from build123d import *

# Parameters (mm, degrees)
F0_R      = 25.4
F1_DEPTH  = 76.2
F2_R      = 9.525
F3_DEPTH  = 19.05
F4_R      = 5.08
F5_SIZE   = 1.27
F6_W      = 19.05
F6_H      = 19.05
F7_DEPTH  = 19.05
F8_R      = 6.931889
F9_DEPTH  = 9.525
F10_R     = 4.338824
F11_DEPTH = 25.4
F12_SIZE  = 1.27
F13_R     = 1.27


with BuildPart() as f1:
    # F0 (on Top) → F1 (new body)
    with BuildSketch(Plane.XY):
        Circle(F0_R)
    extrude(amount=F1_DEPTH)

    # F2 (on face) → F3 (join)
    with BuildSketch(Plane(origin=(0, 0, 0), x_dir=(1, 0, 0), z_dir=(0, 0, -1))):
        Circle(F2_R)
    extrude(amount=F3_DEPTH)

    # F4
    f4_edges = [f1.edges().sort_by_distance(p)[0] for p in [
        (-25.4, 0, 76.2),
    ]]
    fillet(f4_edges, radius=F4_R)

    # F5
    f5_edges = [f1.edges().sort_by_distance(p)[0] for p in [
        (-9.525, 0, -19.05),
    ]]
    chamfer(f5_edges, length=F5_SIZE)

    # F6 (on face) → F7 (join)
    with BuildSketch(Plane.XY.offset(76.2)):
        Rectangle(F6_W, F6_H)
    extrude(amount=F7_DEPTH)

    # F8 (on face) → F9 (join)
    with BuildSketch(Plane.YZ.offset(9.525)):
        with Locations((0, 85.725)):
            Circle(F8_R)
    extrude(amount=F9_DEPTH)

    # F10 (on face) → F11 (cut)
    with BuildSketch(Plane.YZ.offset(19.05)):
        with Locations((0, 85.725)):
            Circle(F10_R)
    extrude(amount=-F11_DEPTH, mode=Mode.SUBTRACT)

    # F12
    f12_edges = [f1.edges().sort_by_distance(p)[0] for p in [
        (0, -9.525, 95.25),
        (-9.525, -9.525, 85.725),
        (9.525, -9.525, 85.725),
        (-9.525, 9.525, 85.725),
        (-9.525, 0, 95.25),
        (9.525, 9.525, 85.725),
        (0, 9.525, 95.25),
        (9.525, 0, 95.25),
    ]]
    chamfer(f12_edges, length=F12_SIZE)

    # F13
    f13_edges = [f1.edges().sort_by_distance(p)[0] for p in [
        (19.05, -6.931889, 85.725),
    ]]
    fillet(f13_edges, radius=F13_R)


solid = f1.part
Geometry check sheet. Reference: the model listing, model coordinates, mm. A direction names the side the tool comes from. Round coordinates to 2 decimals unless told otherwise and drop trailing zeros. Order: outer loops, then holes, each group sorted by start corner. A loop starts at its lowest first (then second) coordinate and runs counter-clockwise, first axis right, second up. Notation, with made-up numbers: M 60.25,69.5 L 93.25,69.5 A12 cw 93.25,76.5 Z; hole C -19,-14.75 d8. An arc over 180 degrees is marked long. Answer in a Markdown table with one row per item.
(1) Tool access check on faces 1 (the face through (9.525, -6, 81)), 2 (the face through (19.05, 3, 82)), 3 (the face through (11, 0, 0)). Record the directions out of +Z, -Z, +X, -X, +Y, -Y that give a thin tool (end or side, any length) a straight path to the whole face; none if there is none.
Responses:
| item | result |
|---|---|
| face 1 | +X |
| face 2 | +Z, +X, +Y, -Y |
| face 3 | -Z |
(2) Sectioned sample at A-A, the plane y = 0. Record the cut outline in (x, z) (3 decimals), and give its area (3 significant figures).
Responses:
| item | result |
|---|---|
| outline | M -25.4,0 L -9.525,0 L -9.525,-17.78 L -8.255,-19.05 L 8.255,-19.05 L 9.525,-17.78 L 9.525,0 L 25.4,0 L 25.4,71.12 A5.08 ccw 20.32,76.2 L 9.525,76.2 L 9.525,78.793 L 17.78,78.793 A1.27 ccw 19.05,80.063 L 19.05,81.386 L -6.35,81.386 L -6.35,90.064 L 19.05,90.064 L 19.05,91.387 A1.27 ccw 17.78,92.657 L 9.525,92.657 L 9.525,93.98 L 8.255,95.25 L -8.255,95.25 L -9.525,93.98 L -9.525,76.2 L -20.32,76.2 A5.08 ccw -25.4,71.12 Z |
| area | 4,490 mm² |
(3) Go/stop test with flat-tipped pins: P1, Ø18, axis at y = -3, z = 81.5, coming from the +X side; P2, Ø10, axis at x = -5.5, z = 18.5, coming from the +Y side; P3, Ø7, axis at y = 0, z = 85.725, coming from the +X side; P4, Ø1.5, axis at x = -20, y = -17, coming from the -Z side. Record where each tip stops, or that it passes through.
Responses:
| item | result |
|---|---|
| P1 | stops at x = 25.13 |
| P2 | stops at y = 25.4 |
| P3 | stops at x = -6.35 |
| P4 | passes through |
(4) Sectioned sample at B-B, the plane x = 0. Record the cut outline in (y, z) (3 decimals), and give its area (3 significant figures).
Responses:
| item | result |
|---|---|
| outline | M -25.4,0 L -9.525,0 L -9.525,-17.78 L -8.255,-19.05 L 8.255,-19.05 L 9.525,-17.78 L 9.525,0 L 25.4,0 L 25.4,71.12 A5.08 ccw 20.32,76.2 L 9.525,76.2 L 9.525,93.98 L 8.255,95.25 L -8.255,95.25 L -9.525,93.98 L -9.525,76.2 L -20.32,76.2 A5.08 ccw -25.4,71.12 Z; hole C 0,85.725 d8.678 |
| area | 4,520 mm² |
(5) Scan lines: probe 1 along Z at (x, y) = (12.5, 0); probe 2 along Z at (x, y) = (0, 0); probe 3 along Z at (x, y) = (14, -1). Record each from-to range of solid material in increasing order. Write a range as from..to.
Responses:
| item | result |
|---|---|
| probe 1 | z = 0..76.2, 78.79..81.39, 90.06..92.66 |
| probe 2 | z = -19.05..81.39, 90.06..95.25 |
| probe 3 | z = 0..76.2, 78.87..81.5, 89.95..92.58 |
(6) Sectioned sample at D-D, the plane z = -4. Record the cut outline in (x, y) (3 decimals).
Responses:
| item | result |
|---|---|
| outline | C 0,0 d19.05 |
(7) Draft check along Y on faces 4 (the face through (-9.525, 0, 85)), 5 (the face through (13.6, -0.9, 92.6)), 6 (the face through (-6.35, 0, 86)). Enter one of: released by +Y, released by -Y, zero draft, split by the parting line, or undercut.
Responses:
| item | result |
|---|---|
| face 4 | zero draft |
| face 5 | split by the parting line |
| face 6 | undercut |
(8) Sectioned sample at C-C, the plane x = 12. State how many separate pieces and enclosed holes the cut face has, and give its area (3 significant figures).
Responses:
| item | result |
|---|---|
| separate pieces | 2 |
| enclosed holes | 1 |
| area | 3,490 mm² |
